```python
from build123d import *

# Parameters (mm, degrees)
SKETCH1_W            = 155
SKETCH1_H            = 285.39
BOSS_EXTRUDE1_DEPTH  = 2.305
M5_CLEARANCE_HOLE1_D = 5.5
SKETCH4_R            = 2.15
SKETCH4_R_2          = 3.25
CUT_EXTRUDE1_DEPTH   = 3.305
SKETCH5_W            = 41
SKETCH5_H            = 13
CUT_EXTRUDE2_DEPTH   = 10
CUT_EXTRUDE3_DEPTH   = 3.305


with BuildPart() as part:
    # Sketch1 → Boss-Extrude1 (new body)
    with BuildSketch(Plane.XY):
        Rectangle(SKETCH1_W, SKETCH1_H)
    extrude(amount=BOSS_EXTRUDE1_DEPTH)

    # M5 Clearance Hole1 (through all)
    with Locations(Plane.XY.offset(2.305)):
        with Locations((-62, 129.995), (0, 129.995), (-62, -129.995), (0, -129.995), (62, -129.995)):
            Hole(M5_CLEARANCE_HOLE1_D / 2)

    # Sketch4 → Cut-Extrude1 (cut, through all)
    with BuildSketch(Plane.XY.offset(2.305)):
        with Locations((30.1, -81)):
            Circle(SKETCH4_R)
        with Locations((42.1, -93)):
            Circle(SKETCH4_R)
        with Locations((30.1, -105)):
            Circle(SKETCH4_R)
        with Locations((18.1, -93)):
            Circle(SKETCH4_R)
        with Locations((30.1, 93)):
            Circle(SKETCH4_R_2)
    extrude(amount=-CUT_EXTRUDE1_DEPTH, mode=Mode.SUBTRACT)

    # Sketch5 → Cut-Extrude2 (cut)
    with BuildSketch(Plane.XY.offset(2.305)):
        with Locations((57, 136.195)):
            Rectangle(SKETCH5_W, SKETCH5_H)
    extrude(amount=-CUT_EXTRUDE2_DEPTH, mode=Mode.SUBTRACT)

    # Sketch6 → Cut-Extrude3 (cut, through all)
    with BuildSketch(Plane.XY.offset(2.305)):
        with BuildLine():
            Line((26.5, 65), (50.5, 65))
            Line((50.5, 65), (50.5, -65))
            Line((50.5, -65), (26.5, -65))
            Line((26.5, -65), (26.5, -15))
            ThreePointArc((26.5, -15), (11.5, 0), (26.5, 15))
            Line((26.5, 15), (26.5, 65))
        make_face()
    extrude(amount=-CUT_EXTRUDE3_DEPTH, mode=Mode.SUBTRACT)


solid = part.part
```
Geometry check sheet. Reference: the model listing, model coordinates, mm. Round coordinates to 2 decimals unless told otherwise and drop trailing zeros. Order: outer loops, then holes, each group sorted by start corner. A loop starts at its lowest first (then second) coordinate and runs counter-clockwise, first axis right, second up. Notation, with made-up numbers: (25, 27) - (63, 27) arc R15 ccw to (63, 45) - close; hole circle Ø10 at (-15.5, -32.5). An arc over 180 degrees is marked (long way). Use a Markdown table: item, result. Add a question column.
1) Mould release check, pull along X, two halves, no side actions. Record for faces 1 (the cylindrical face through (29.395, 89.827, 1.169)), 2 (the flat face through (-1, 2, 0)), 3 (the cylindrical face through (11.504, -0.33, 1.169)): released by +X, released by -X, zero draft, split by the parting line, or undercut.
2) Section check A-A (y = 0). Record the cut outline in (x, z) (3 decimals), then the cut area to 3 significant figures.
3) Section check C-C (y = 44). Record the cut outline in (x, z) (3 decimals), then the cut area to 3 significant figures.
4) Section check B-B (x = -62). Record the cut outline in (y, z) (3 decimals).
5) Thickness scan on line 1 along Y through (x, z) = (42.1, 1.2) (3 decimals); line 2 along X through (y, z) = (130.5, 1.95); line 3 along Y through (x, z) = (30.1, 1.1) (3 decimals). Record the ranges inside material, lowest first.
Established:
| question | item | result |
|---|---|---|
| 1 | face 1 | undercut |
| 1 | face 2 | zero draft |
| 1 | face 3 | undercut |
| 2 | outline | (-77.5, 0) - (11.5, 0) - (11.5, 2.305) - (-77.5, 2.305) - close; (50.5, 0) - (77.5, 0) - (77.5, 2.305) - (50.5, 2.305) - close |
| 2 | area | 267 mm2 |
| 3 | outline | (-77.5, 0) - (26.5, 0) - (26.5, 2.305) - (-77.5, 2.305) - close; (50.5, 0) - (77.5, 0) - (77.5, 2.305) - (50.5, 2.305) - close |
| 3 | area | 302 mm2 |
| 4 | outline | (-142.695, 0) - (-132.745, 0) - (-132.745, 2.305) - (-142.695, 2.305) - close; (-127.245, 0) - (127.245, 0) - (127.245, 2.305) - (-127.245, 2.305) - close; (132.745, 0) - (142.695, 0) - (142.695, 2.305) - (132.745, 2.305) - close |
| 5 | line 1 | -142.695 to -95.15, -90.85 to -65, 65 to 129.695 |
| 5 | line 2 | -77.5 to -64.7, -59.3 to -2.7, 2.7 to 36.5 |
| 5 | line 3 | -142.695 to -107.15, -102.85 to -83.15, -78.85 to -65, 65 to 89.75, 96.25 to 142.695 |
